The listing builds one solid part. Answer for the finished solid, in the listing's coordinates (mm). Coordinates: 2 decimals unless noted, no trailing zeros. Write each loop counter-clockwise with the first axis right and the second up, starting at its lowest first coordinate (ties: lowest second). Pieces come first, ordered by that corner, then holes.
Autodesk Inventor part; units mm, degrees
ref_plane "YZ Plane" through (0, 0, 0) normal (1, 0, 0) x (0, 1, 0)
ref_plane "XZ Plane" through (0, 0, 0) normal (0, 1, 0) x (-1, 0, 0)
ref_plane "XY Plane" through (0, 0, 0) normal (0, 0, 1) x (1, 0, 0)
sketch "Sketch1" plane through (0, 0, 0) normal (0, 0, 1) x (1, 0, 0)
  line L0 (-13.3, 8.2) -> (13.3, 8.2)
  line L1 (13.3, 8.2) -> (13.3, -8.2)
  line L2 (13.3, -8.2) -> (-13.3, -8.2)
  line L3 (-13.3, -8.2) -> (-13.3, 8.2)
  point P0 (0, 0)
  point P1 (-13.3, 0)
  point P2 (0, 8.2)
  dimension "d0" = 26.6
  dimension "d1" = 16.4
extrude "Extrusion1" add sketch "Sketch1" along normal blind 2
sketch "Sketch2" plane through (0, 0, 2) normal (0, 0, 1) x (1, 0, 0)
  circle A0 centre (-10.5, 0) radius 1.5
  circle A1 centre (10.5, 0) radius 1.5
  point P0 (0, 0)
  dimension "d4" = 3
  dimension "d5" = 21
  dimension "d6" = 10.5
hole "Hole1" at (10.5, 0, 2) direction (0, 0, -1) diameter 3.5 end through all
pattern_linear "Rectangular Pattern1" count 2 spacing 21 along (-1, 0, 0) of "Hole1"
equation "\"d16\" = d5"
properties part number "LogicLevelConverter" material "PET Plastic"
Q1. The part is cut by section B-B, the plane y = 0. Write down the section's boundary in (x, z).
Answers below:
outline: (-13.3, 0) - (-12.25, 0) - (-12.25, 2) - (-13.3, 2) - close; (-8.75, 0) - (8.75, 0) - (8.75, 2) - (-8.75, 2) - close; (12.25, 0) - (13.3, 0) - (13.3, 2) - (12.25, 2) - close
Q2. Determine the mould class of faces 1 (the face through (0, -8.2, 1)), 2 (the face through (0, 0, 0)), 3 (the face through (8.765, 0.228, 0.986)) for opening direction Y: released by +Y, released by -Y, zero draft, split by the parting line, or undercut.
Answers below:
face 1: released by -Y
face 2: zero draft
face 3: undercut
Q3. Given pin 1 (1.5 mm diameter, centred on x = 10, y = -2, fed in from -Z); pin 2 (3 mm diameter, centred on x = -10.5, y = 0, fed in from +Z), each flat-ended and moving along its own axis, determine where each tip first touches the part or whether it passes through.
Answers below:
pin 1: stops at z = 0
pin 2: passes through
Q4. The part is cut by section C-C, the plane z = 0.7. Write down the section's boundary in (x, y), then the cut area to 3 significant figures.
Answers below:
outline: (-13.3, -8.2) - (13.3, -8.2) - (13.3, 8.2) - (-13.3, 8.2) - close; hole circle Ø3.5 at (-10.5, 0); hole circle Ø3.5 at (10.5, 0)
area: 417 mm2
Q5. Find the intervals of material crossed by probe 1 along X at (y, z) = (0, 0.95); probe 2 along Y at (x, z) = (10.5, 0.55); probe 3 along X at (y, z) = (1, 1.65), in increasing order.
Answers below:
probe 1: x = -13.3 to -12.25, -8.75 to 8.75, 12.25 to 13.3
probe 2: y = -8.2 to -1.75, 1.75 to 8.2
probe 3: x = -13.3 to -11.94, -9.06 to 9.06, 11.94 to 13.3
Q6. The part is cut by section A-A, the plane x = 10.5. Write down the section's boundary in (y, z).
Answers below:
outline: (-8.2, 0) - (-1.75, 0) - (-1.75, 2) - (-8.2, 2) - close; (1.75, 0) - (8.2, 0) - (8.2, 2) - (1.75, 2) - close
